```python
from build123d import *

# Parameters (mm, degrees)
SKETCH_1_R      = 2
EXTRUDE_1_DEPTH = 3
FILLET_1_R      = 3


with BuildPart() as part:
    # 草图1 → 凸台-拉伸1 (new body)
    with BuildSketch(Plane(origin=(0, 0, 0), x_dir=(1, 0, 0), z_dir=(0, 1, 0))):
        with BuildLine():
            Line((31.622776602, 15), (56.622776602, 15))
            Line((56.622776602, 15), (56.622776602, -15))
            Line((56.622776602, -15), (31.622776602, -15))
            ThreePointArc((31.622776602, -15), (35, 0), (31.622776602, 15))
        make_face()
        with Locations(Location((50, 8, 0), (0, 0, 270))):
            Circle(SKETCH_1_R, mode=Mode.SUBTRACT)
        with Locations(Location((50, -8, 0), (0, 0, 90))):
            Circle(SKETCH_1_R, mode=Mode.SUBTRACT)
    extrude(amount=EXTRUDE_1_DEPTH)

    # 圆角1
    fillet_1_edges = [part.edges().sort_by_distance(p)[0] for p in [
        (56.622776602, 1.5, -15),
        (56.622776602, 1.5, 15),
    ]]
    fillet(fillet_1_edges, radius=FILLET_1_R)


solid = part.part
```
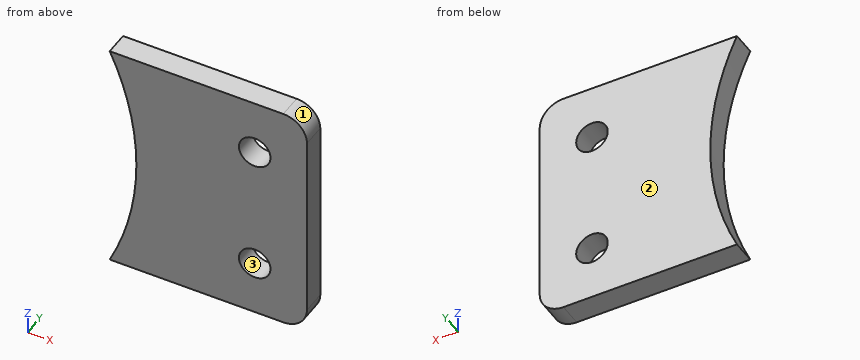
Here's how the part is built. I have some questions about the finished solid (model axes, mm). Face numbers are marked on the shaded views. Give positions to 0.01 mm unless a question says otherwise; leave off trailing zeros. Loops run counter-clockwise (first coordinate to the right, second up) from the corner with the lowest first, then second, coordinate; pieces in that order, holes last. Notation, with made-up numbers: (69.25, -32) -> (84.25, -32) arc R26 ccw to (84.25, -16) -> close; hole circle Ø6 at (12.5, 35.5). An arc over 180 degrees is marked (long way). Use one line per item in the form item = value. Start each with the question number.
1) For P1, Ø1, axis at y = 1.5, z = -11, coming from the -X side, with a flat end and sliding along its axis, tell me the tip position at first contact or that it passes through.
2) Imagine slicing it at D-D (z = -5). Please give me the cut outline in (x, y).
3) Please list where these lines run through material, in increasing order: line 1 along X through (y, z) = (1.3, -9); line 2 along X through (y, z) = (1.1, 8.5); line 3 along X through (y, z) = (2.4, -2).
4) Imagine slicing it at C-C (z = 8). Please give me the cut outline in (x, y).
5) Thinking about a two-plate mould opening in X: for the marked faces 1, 2 and 3, which applies, +X half, -X half, draft (parallel to the pull), parting line (faces both ways), or undercut?
6) Imagine slicing it at A-A (x = 50). Please give me the cut outline in (y, z).
7) Imagine slicing it at B-B (y = 1.5). Please give me the cut outline in (x, z), then the cut area to 3 significant figures.
Check values:
q1.P1 = 33.06
q2.outline = (34.64, 0) -> (56.62, 0) -> (56.62, 3) -> (34.64, 3) -> close
q3.line_1 = 33.82 to 48.27, 51.73 to 56.62
q3.line_2 = 33.95 to 48.06, 51.94 to 56.62
q3.line_3 = 34.94 to 56.62
q4.outline = (34.07, 0) -> (48, 0) -> (48, 3) -> (34.07, 3) -> close; (52, 0) -> (56.62, 0) -> (56.62, 3) -> (52, 3) -> close
q5.face_1 = +X half
q5.face_2 = draft
q5.face_3 = undercut
q6.outline = (0, -15) -> (3, -15) -> (3, -10) -> (0, -10) -> close; (0, -6) -> (3, -6) -> (3, 6) -> (0, 6) -> close; (0, 10) -> (3, 10) -> (3, 15) -> (0, 15) -> close
q7.outline = (31.62, -15) -> (53.62, -15) arc R3 ccw to (56.62, -12) -> (56.62, 12) arc R3 ccw to (53.62, 15) -> (31.62, 15) arc R35 cw to start; hole circle Ø4 at (50, -8); hole circle Ø4 at (50, 8)
q7.area = 653 mm^2
